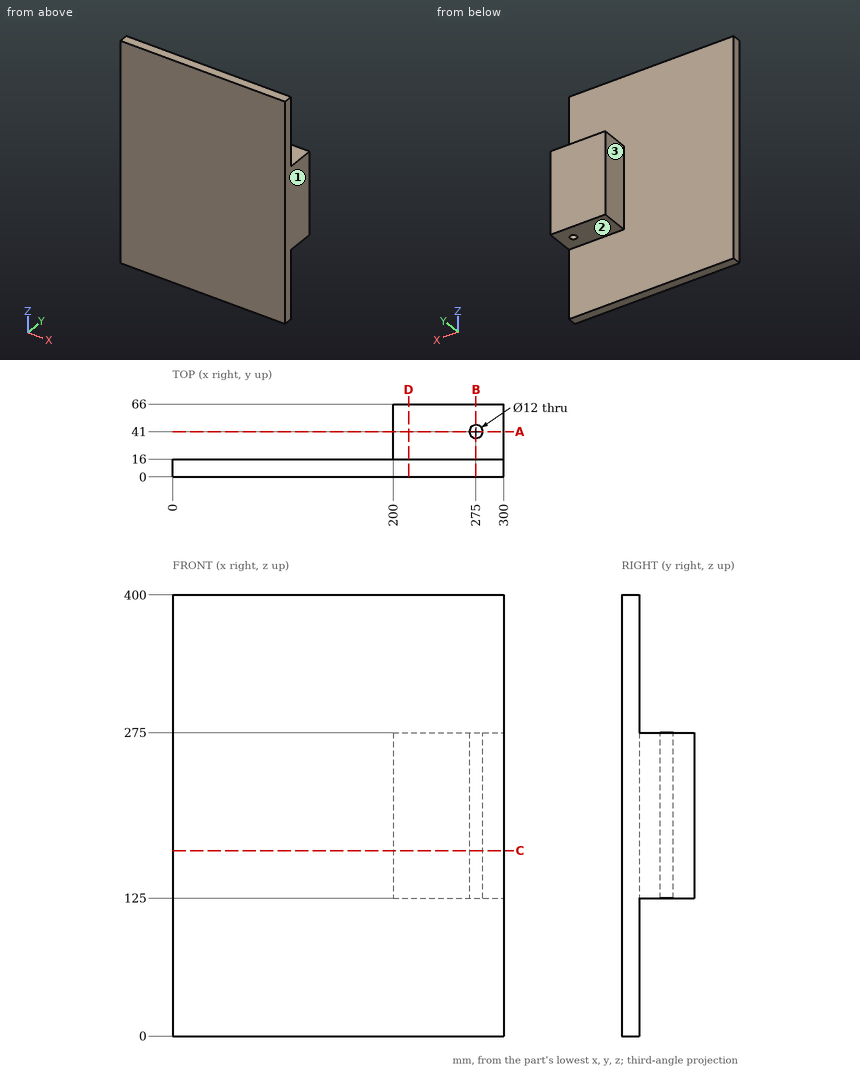
Geometry: see drawing. Coordinates: mm, zero at the bounding-box minimum. A direction names the side the tool comes from. Coordinates: 2 decimals unless noted, no trailing zeros. Order: outer loops, then holes, each group sorted by start corner. A loop starts at its lowest first (then second) coordinate and runs counter-clockwise, first axis right, second up. Notation, with made-up numbers: M -27.5,-34.5 L -4.5,-34.5 A10 ccw -4.5,-23.5 Z; hole C 23.25,45.5 d8. An arc over 180 degrees is marked long. Write item = value, one per line. Start each with the question number.
(1) Section C-C on z = 168. Output: boundary loops of the cut face in (x, y), and give its area (3 significant figures).
(2) Section D-D on x = 214. Output: boundary loops of the cut face in (y, z), and give its area (3 significant figures).
(3) Section B-B on x = 275. Output: boundary loops of the cut face in (y, z), and give its area (3 significant figures).
(4) First-contact query: P1, Ø10, axis at x = 184.5, z = 328, coming from the +Y side; P2, Ø1.5, axis at x = 210, y = 49.5, coming from the +Z side; P3, Ø25, axis at x = 241, y = 50, coming from the -Z side. Flat tips, straight axial feed; report the tip coordinate or a pass-through.
(5) Reachability of the marked faces 1, 2 and 3 from +Z, -Z, +X, -X, +Y, -Y: full face, straight path, thin tool, end or side. Return the list, or none.
(6) Section A-A on y = 41. Output: boundary loops of the cut face in (x, z), and give its area (3 significant figures).
(7) Line query: line 1 along X through (y, z) = (40, 210.5); line 2 along Y through (x, z) = (275, 157); line 3 along X through (y, z) = (41, 239). Output: solid intervals per line, ascending. Write a range as [from, to].
Result set:
q1.outline = M 0,0 L 300,0 L 300,66 L 200,66 L 200,16 L 0,16 Z; hole C 275,41 d12
q1.area = 9,690 mm²
q2.outline = M 0,0 L 16,0 L 16,125 L 66,125 L 66,275 L 16,275 L 16,400 L 0,400 Z
q2.area = 13,900 mm²
q3.outline = M 0,0 L 16,0 L 16,125 L 35,125 L 35,275 L 16,275 L 16,400 L 0,400 Z; M 47,125 L 66,125 L 66,275 L 47,275 Z
q3.area = 12,100 mm²
q4.P1 = 16
q4.P2 = 275
q4.P3 = 125
q5.face_1 = +Z, -Z, +X, +Y, -Y
q5.face_2 = -Z, +X, -X, +Y
q5.face_3 = +Z, -Z, -X, +Y
q6.outline = M 200,125 L 269,125 L 269,275 L 200,275 Z; M 281,125 L 300,125 L 300,275 L 281,275 Z
q6.area = 13,200 mm²
q7.line_1 = [200, 269.08], [280.92, 300]
q7.line_2 = [0, 35], [47, 66]
q7.line_3 = [200, 269], [281, 300]
